Autodesk Inventor part; units mm, degrees
ref_plane "YZ Plane" through (0, 0, 0) normal (1, 0, 0) x (0, 1, 0)
ref_plane "XZ Plane" through (0, 0, 0) normal (0, 1, 0) x (-1, 0, 0)
ref_plane "XY Plane" through (0, 0, 0) normal (0, 0, 1) x (1, 0, 0)
sketch "Boceto1" plane through (0, 0, 0) normal (0, 1, 0) x (-1, 0, 0)
  line L0 (-25.25, 75.25) -> (25.25, 75.25)
  line L1 (25.25, 75.25) -> (25.25, -75.25)
  line L2 (25.25, -75.25) -> (-25.25, -75.25)
  line L3 (-25.25, -75.25) -> (-25.25, 75.25)
  line L4 (-25.25, 75.25) -> (25.25, -75.25) construction
  line L5 (25.25, 75.25) -> (-25.25, -75.25) construction
  line L6 (22.25, -72.25) -> (22.25, 72.25)
  line L7 (22.25, 72.25) -> (-22.25, 72.25)
  line L8 (-22.25, 72.25) -> (-22.25, -72.25)
  line L9 (-22.25, -72.25) -> (22.25, -72.25)
  point P0 (0, 0)
  dimension "d0" = 50.5
  dimension "d1" = 150.5
  dimension "d2" = 3
  dimension "d3" = 44.5
extrude "Extrusión1" add sketch "Boceto1" along normal blind 79
sketch "Boceto2" plane through (0, 79, 0) normal (0, 1, 0) x (1, 0, 0)
  line L0 (-22.25, -72.25) -> (-22.25, 72.25)
  line L1 (25.25, 75.25) -> (-25.25, 75.25)
  line L2 (-25.25, 75.25) -> (-25.25, -75.25)
  line L3 (-25.25, -75.25) -> (25.25, -75.25)
  line L4 (25.25, -75.25) -> (25.25, 75.25)
  line L5 (-22.25, 72.25) -> (22.25, 72.25)
  line L6 (22.25, 72.25) -> (22.25, -72.25)
  line L7 (22.25, -72.25) -> (-22.25, -72.25)
  line L8 (-22.25, -72.25) -> (-22.25, 72.25)
  point P0 (0, 0)
  point P1 (-22.25, 72.25)
extrude "Extrusión2" add sketch "Boceto2" against normal blind 3 contours L0 L5 L6 L7
fillet "Empalme1" radius 1 4 edges at (0, 79, 75.25) (25.25, 79, 0) (-25.25, 79, 0) (0, 79, -75.25)
sketch "Boceto3" plane through (0, 0, 0) normal (0, -1, 0) x (1, 0, 0)
  line L0 (25.25, -75.25) -> (-25.25, -75.25)
  line L1 (25.25, 75.25) -> (25.25, -75.25)
  line L2 (-25.25, 75.25) -> (25.25, 75.25)
  line L3 (-25.25, -75.25) -> (-25.25, 75.25)
  line L4 (-22.25, -72.25) -> (22.25, -72.25)
  line L5 (-22.25, 72.25) -> (-22.25, -72.25)
  line L6 (22.25, 72.25) -> (-22.25, 72.25)
  line L7 (22.25, -72.25) -> (22.25, 72.25)
  line L8 (23.85, 73.85) -> (-23.85, 73.85)
  line L9 (-23.85, 73.85) -> (-23.85, -73.85)
  line L10 (-23.85, -73.85) -> (23.85, -73.85)
  line L11 (23.85, -73.85) -> (23.85, 73.85)
  point P0 (0, 0)
  dimension "d9" = 1.6
extrude "Extrusión3" add sketch "Boceto3" along normal blind 8 contours L11 L10 L9 L8
fillet "Empalme2" radius 1.6 4 edges at (-23.85, -8, 0) (0, -8, 73.85) (23.85, -8, 0) (0, -8, -73.85)
fillet "Empalme3" radius 1.6 4 edges at (22.25, 76, 0) (0, 76, 72.25) (0, 76, -72.25) (-22.25, 76, 0)
fillet "Empalme4" radius 1.6 16 edges at (-24.9571, 78.7071, 74.9571) (-25.25, 39, 75.25) (24.9571, 78.7071, 74.9571) (25.25, 39, 75.25) (-24.9571, 78.7071, -74.9571) (-25.25, 39, -75.25) (24.9571, 78.7071, -74.9571) (25.25, 39, -75.25) (-23.3814, -7.5314, -73.3814) (-23.85, -3.2001, -73.85) (23.3814, -7.5314, -73.3814) (23.85, -3.2001, -73.85) (-23.3814, -7.5314, 73.3814) (-23.85, -3.2001, 73.85) (23.3814, -7.5314, 73.3814) (23.85, -3.2001, 73.85)
properties part number "Caja bateria"
Input: part model. Units: mm. Frame: model coordinates. A direction names the side the tool comes from. Give positions to 0.01 mm unless a question says otherwise; leave off trailing zeros. Order: outer loops, then holes, each group sorted by start corner. A loop starts at its lowest first (then second) coordinate and runs counter-clockwise, first axis right, second up. Notation, with made-up numbers: M 6.25,21 L 22.25,21 A20 cw 22.25,51 Z; hole C 11.25,36 d1. An arc over 180 degrees is marked long. Return JSON: item names as keys, results as strings.
Item 1: Pull-direction query (X, two-part tool) for faces 1 (the flat face through (0, 38, -75.25)), 2 (the flat face through (25.25, 38, -1)), 3 (the flat face through (0, 76, -1)); classes: +X half, -X half, draft (parallel to the pull), parting line (faces both ways), or undercut.
Solutions:
{"face 1": "draft", "face 2": "+X half", "face 3": "undercut"}
Item 2: Cut plane A-A (y = 5.5). Return loops of the section in (x, z), then the cut area to 3 significant figures.
Solutions:
{"outline": "M -25.25,-73.65 A1.6 ccw -23.65,-75.25 L 23.65,-75.25 A1.6 ccw 25.25,-73.65 L 25.25,73.65 A1.6 ccw 23.65,75.25 L -23.65,75.25 A1.6 ccw -25.25,73.65 Z; hole M -22.25,-72.25 L 22.25,-72.25 L 22.25,72.25 L -22.25,72.25 Z", "area": "1,170 mm^2"}
Item 3: Access query for faces 4 (the flat face through (0, -3, -73.85)), 5 (the flat face through (23.85, -3, -1)), 6 (the flat face through (22.25, 34, -1)). Directions: +Z, -Z, +X, -X, +Y, -Y. A direction counts if a zero-diameter tool reaches every point of the face in a straight line with its end or side. Return the directions, or none.
Solutions:
{"face 4": "-Z, +X, -X, -Y", "face 5": "+Z, -Z, +X, -Y", "face 6": "-Y"}
Item 4: Ray query, probe 1 along Z at (x, y) = (-7.5, 43); probe 2 along X at (y, z) = (66, 22); probe 3 along Y at (x, z) = (15.5, 5). Return the intervals inside material, ascending.
Solutions:
{"probe 1": "-75.25 to -72.25, 72.25 to 75.25", "probe 2": "-25.25 to -22.25, 22.25 to 25.25", "probe 3": "76 to 79"}
Item 5: First-contact query: P1, Ø3, axis at y = -3, z = -24, coming from the +X side; P2, Ø3, axis at x = 1, y = -3.5, coming from the -Z side; P3, Ø5, axis at x = 2.5, y = -3.5, coming from the +Z side. Flat tips, straight axial feed; report the tip coordinate or a pass-through.
Solutions:
{"P1": "x = 23.85", "P2": "z = -73.85", "P3": "z = 73.85"}
